Input: dimensioned drawing with shaded views. Units: mm. Origin: part minimum x, y, z. Give positions to 0.01 mm unless a question says otherwise; leave off trailing zeros. Write each loop counter-clockwise with the first axis right and the second up, starting at its lowest first coordinate (ties: lowest second). Pieces come first, ordered by that corner, then holes.
Q1. Section B-B (y = 0.65). State how many separate pieces and enclosed holes the cut face has, plus the area to 3 significant figures.
Q2. Line query: line 1 (X direction, y = 1.6, z = 31.75) (3 decimals); line 2 (Z direction, x = 78.74, y = 1.25) (3 decimals); line 3 (Z direction, x = 14, y = 2.1) (3 decimals). Output: solid intervals per line, ascending.
Q3. Section C-C (x = 12.7). Return the cut outline in (y, z) (3 decimals), plus the area to 3 significant figures.
Q4. Section A-A (z = 106.04). Return the cut outline in (x, y), plus the area to 3 significant figures.
Q5. Pin query (flat end, axial travel): pin 1 Ø2 at (x, z) = (28.525, 106.04) entering from -Y. Return the tip coordinate at first contact, or that it passes through.
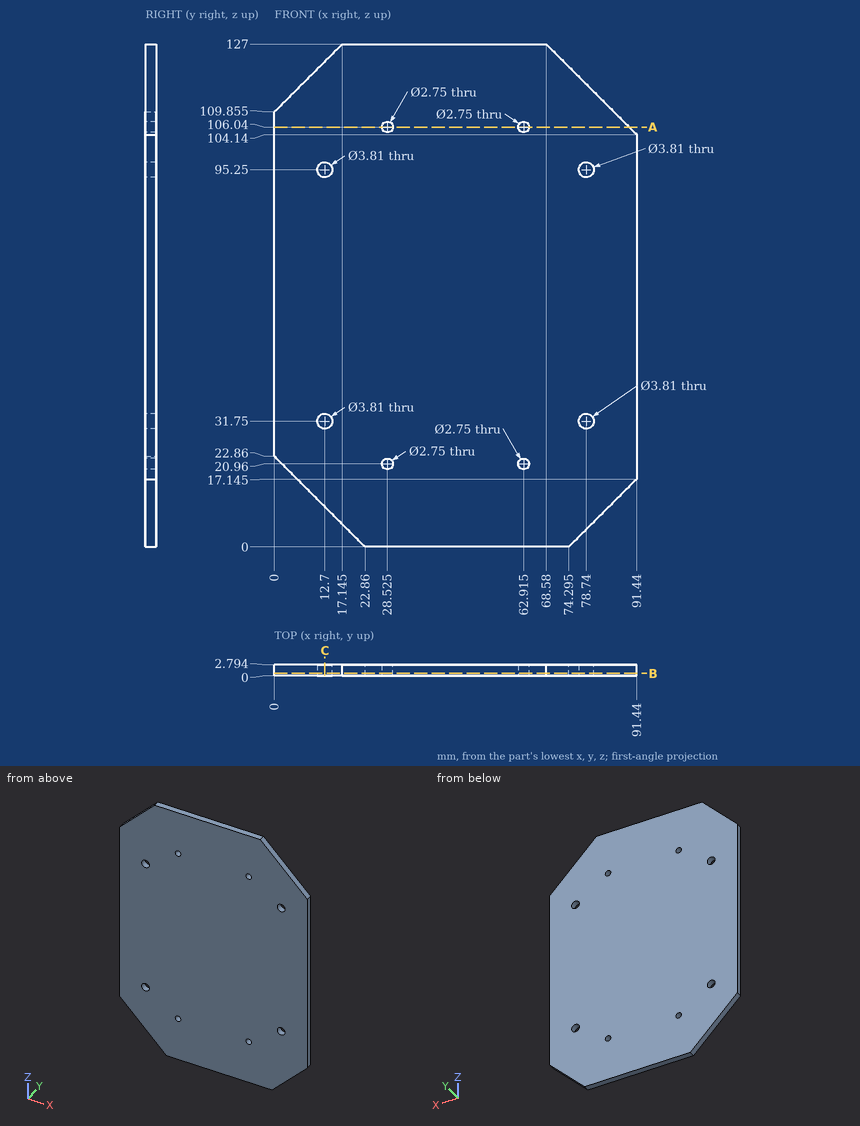
Computed:
1. separate pieces: 1
1. enclosed holes: 8
1. area: 10,700 mm2
2. line 1: x = 0 to 10.795, 14.605 to 76.835, 80.645 to 91.44
2. line 2: z = 4.445 to 29.845, 33.655 to 93.345, 97.155 to 116.84
2. line 3: z = 8.86 to 30.358, 33.142 to 93.858, 96.642 to 123.855
3. outline: (0, 10.16) - (2.794, 10.16) - (2.794, 29.845) - (0, 29.845) - close; (0, 33.655) - (2.794, 33.655) - (2.794, 93.345) - (0, 93.345) - close; (0, 97.155) - (2.794, 97.155) - (2.794, 122.555) - (0, 122.555) - close
3. area: 293 mm2
4. outline: (0, 0) - (27.15, 0) - (27.15, 2.79) - (0, 2.79) - close; (29.9, 0) - (61.54, 0) - (61.54, 2.79) - (29.9, 2.79) - close; (64.29, 0) - (89.54, 0) - (89.54, 2.79) - (64.29, 2.79) - close
4. area: 235 mm2
5. pin 1: passes through
